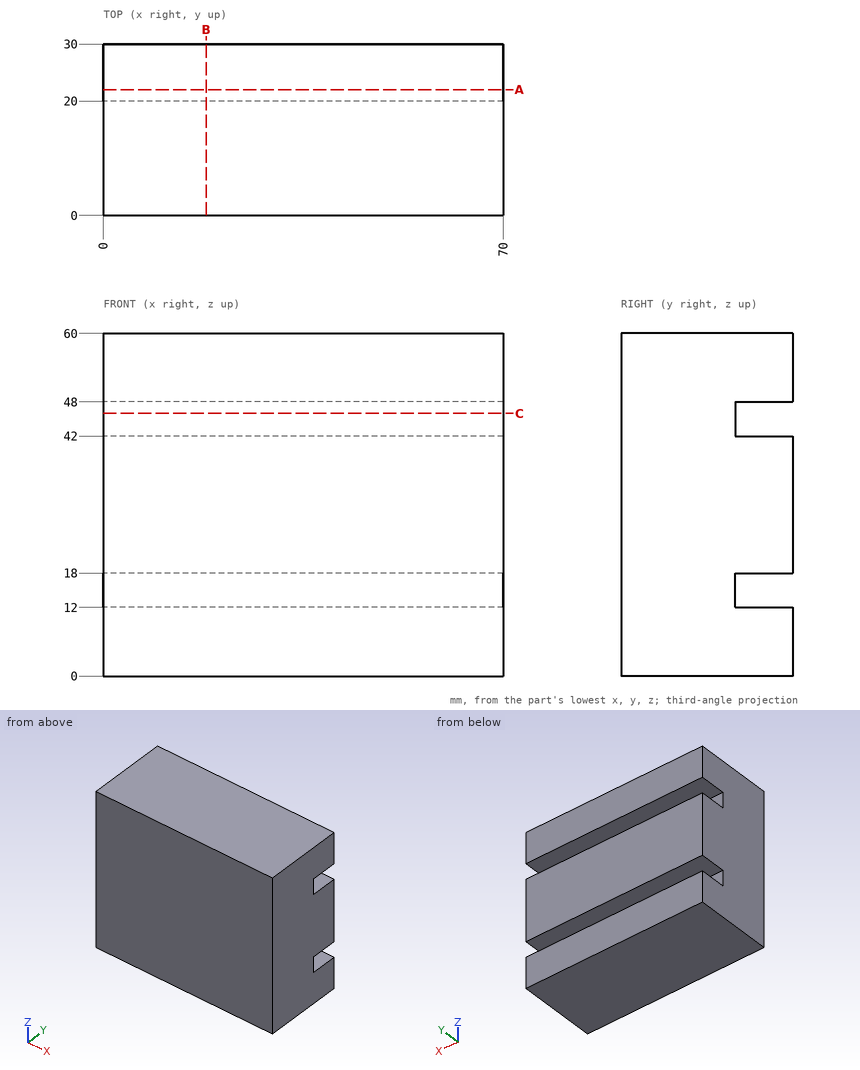
Geometry check sheet. Reference: drawing and pictorial views, mm from the part's lowest x, y, z. Coordinates: 2 decimals unless noted, no trailing zeros. Order: outer loops, then holes, each group sorted by start corner. A loop starts at its lowest first (then second) coordinate and runs counter-clockwise, first axis right, second up.
Item 1: Depth check by flat-ended pin: pin 1 (5 mm diameter, centred on x = 33, z = 45, fed in from +Y). Enter the tip coordinate at first touch or a pass-through.
Item 2: Section check B-B (x = 18). Enter the section's corners in (y, z), plus the area to 3 significant figures.
Item 3: Section check A-A (y = 22). Enter the section's corners in (x, z), plus the area to 3 significant figures.
Item 4: Section check C-C (z = 46). Enter the section's corners in (x, y).
Item 5: Scan lines: line 1 along Z through (x, y) = (13, 23); line 2 along Y through (x, z) = (63, 44.5). Record each from-to range of solid material in increasing order.
Check sheet entries:
1. pin 1: stops at y = 20
2. outline: (0, 0) - (30, 0) - (30, 12) - (20, 12) - (20, 18) - (30, 18) - (30, 42) - (20, 42) - (20, 48) - (30, 48) - (30, 60) - (0, 60) - close
2. area: 1,680 mm2
3. outline: (0, 0) - (70, 0) - (70, 12) - (0, 12) - close; (0, 18) - (70, 18) - (70, 42) - (0, 42) - close; (0, 48) - (70, 48) - (70, 60) - (0, 60) - close
3. area: 3,360 mm2
4. outline: (0, 0) - (70, 0) - (70, 20) - (0, 20) - close
5. line 1: z = 0 to 12, 18 to 42, 48 to 60
5. line 2: y = 0 to 20
